from build123d import *

# Parameters (mm, degrees)
SKETCH1_R           = 7.499999986
BOSS_EXTRUDE1_DEPTH = 22
SKETCH2_W           = 39
SKETCH2_H           = 180
BOSS_EXTRUDE2_DEPTH = 25
FILLET1_R           = 10


with BuildPart() as part:
    # Sketch1 → Boss-Extrude1 (new body)
    with BuildSketch(Plane(origin=(0, 0, 0), x_dir=(0, 0, -1), z_dir=(1, 0, 0))):
        Circle(SKETCH1_R)
    extrude(amount=BOSS_EXTRUDE1_DEPTH)

    # Sketch2 → Boss-Extrude2 (add)
    with BuildSketch(Plane(origin=(22, 0, 0), x_dir=(0, 0, -1), z_dir=(1, 0, 0))):
        Rectangle(SKETCH2_W, SKETCH2_H)
    extrude(amount=BOSS_EXTRUDE2_DEPTH)

    # Fillet1
    fillet1_edges = [part.edges().sort_by_distance(p)[0] for p in [
        (22, 0, 19.5),
        (22, -90, 0),
        (22, 90, 0),
        (47, 0, 19.5),
        (47, -90, 0),
        (47, 90, 0),
    ]]
    fillet(fillet1_edges, radius=FILLET1_R)


solid = part.part
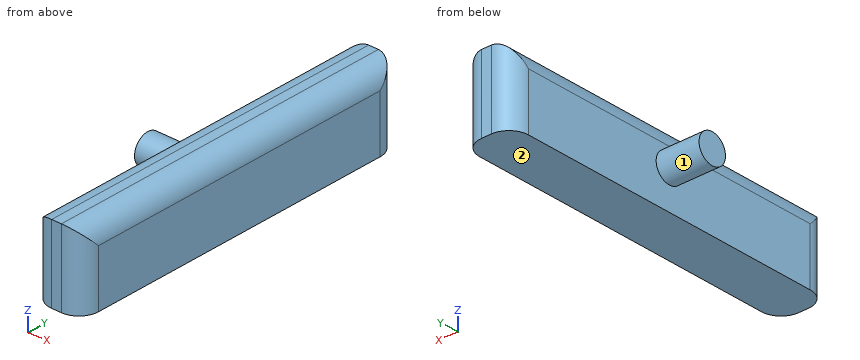
Build history of the part. All positions in model axes, mm. Face numbers are marked on the shaded views. A direction names the side the tool comes from. Coordinates: 2 decimals unless noted, no trailing zeros. Order: outer loops, then holes, each group sorted by start corner. A loop starts at its lowest first (then second) coordinate and runs counter-clockwise, first axis right, second up. Notation, with made-up numbers: M -7,-35 L 48,-35 A15 cw 48,-14 Z; hole C -7,72 d9. An arc over 180 degrees is marked long. One line per question, with ' | ' between items. Start each with the question number.
Q1. Saw through at C-C (x = 11.5). List the corners of the cut face in (y, z).
Q2. 3-axis set-ups, long thin cutter, end or side, ignore diameter. For the marked faces 1 and 2: which of +Z, -Z, +X, -X, +Y, -Y reach the whole face in a straight line?
Q3. Flat gauge pins, fed straight in: pin 1 Ø8 at (x, y) = (15, -57.5) entering from -Z; pin 2 Ø1 at (y, z) = (-43, 11) entering from -X; pin 3 Ø12 at (x, z) = (6.5, 6.5) entering from +Y; pin 4 Ø3 at (x, z) = (40.5, -10) entering from -Y. Where does each tip first touch, or does it go through?
Q4. Saw through at A-A (y = 0). List the corners of the cut face in (x, z), then the cut area to 3 significant figures.
Q5. Saw through at D-D (y = -49). List the corners of the cut face in (x, z).
Q6. Probe L1, parallel to X at y = 55.5, z = -11; L2, parallel to Y at x = 44, z = 13; L3, parallel to Y at x = 23, z = -7. List the from-to ranges inside material, lowest first. Write a range as from..to.
Q7. Saw through at B-B (z = -10.5). List the corners of the cut face in (x, y), then the cut area to 3 significant figures.
Check values:
1) outline: C 0,0 d15
2) face 1: -X | face 2: -Z, +X, -X, +Y, -Y
3) pin 1: passes through | pin 2: stops at x = 22.05 | pin 3: stops at y = 7.48 | pin 4: stops at y = -89.8
4) outline: M 0,-7.5 L 22,-7.5 L 22,-19.5 L 47,-19.5 L 47,9.5 A10 ccw 37,19.5 L 32,19.5 A10 ccw 22,9.5 L 22,7.5 L 0,7.5 Z | area: 1,260 mm2
5) outline: M 22,-19.5 L 47,-19.5 L 47,9.5 A10 ccw 37,19.5 L 32,19.5 A10 ccw 22,9.5 Z
6) L1: x = 22..47 | L2: y = -87.14..87.14 | L3: y = -84.36..84.36
7) outline: M 22,-80 A10 ccw 32,-90 L 37,-90 A10 ccw 47,-80 L 47,80 A10 ccw 37,90 L 32,90 A10 ccw 22,80 Z | area: 4,410 mm2
